from build123d import *

# Parameters (mm, degrees)
F0_R     = 8
F1_DEPTH = 3.5
F2_R     = 12.5
F2_R_2   = 8
F3_DEPTH = 1
F4_W     = 1.5
F4_H     = 2
F4_W_2   = 2
F4_H_2   = 1.5
F5_DEPTH = 0.25
F6_W     = 20
F6_H     = 2
F7_DEPTH = 1.5


with BuildPart() as f1:
    # F0 (on Top) → F1 (new body)
    with BuildSketch(Plane.XY):
        with BuildLine():
            ThreePointArc((0, -12.5), (8.838835, -8.838835), (12.5, 0))
            ThreePointArc((12.5, 0), (8.838835, 8.838835), (0, 12.5))
            ThreePointArc((0, 12.5), (-12.5, 0), (0, -12.5))
        make_face()
        Circle(F0_R, mode=Mode.SUBTRACT)
        with BuildLine():
            ThreePointArc((0, 12.5), (8.838835, 8.838835), (12.5, 0))
            ThreePointArc((12.5, 0), (8.838835, -8.838835), (0, -12.5))
            Line((0, -12.5), (35, -12.5))
            Line((35, -12.5), (116.388784, -2.506714))
            Line((116.388784, -2.506714), (116.388784, 2.506714))
            Line((116.388784, 2.506714), (35, 12.5))
            Line((35, 12.5), (0, 12.5))
        make_face()
    extrude(amount=F1_DEPTH)

    # F2 (on face) → F3 (join)
    with BuildSketch(Plane.XY.offset(3.5)):
        Circle(F2_R)
        Circle(F2_R_2, mode=Mode.SUBTRACT)
    extrude(amount=F3_DEPTH)

    # F4 (on face) → F5 (join)
    with BuildSketch(Plane.XY.offset(4.5)):
        with Locations((0, 10)):
            Rectangle(F4_W, F4_H)
        Polygon((-2.685895, 10.693384), (-4.112479, 10.229859), (-3.494445, 8.327746), (-2.067861, 8.791271), align=None)
        Polygon((-5.858875, 9.340026), (-7.072401, 8.458348), (-5.89683, 6.840314), (-4.683305, 7.721992), align=None)
        Polygon((-8.458348, 7.072401), (-9.340026, 5.858875), (-7.721992, 4.683305), (-6.840314, 5.89683), align=None)
        Polygon((-10.229859, 4.112479), (-10.693384, 2.685895), (-8.791271, 2.067861), (-8.327746, 3.494445), align=None)
        with Locations((-10, 0)):
            Rectangle(F4_W_2, F4_H_2)
        Polygon((-10.693384, -2.685895), (-10.229859, -4.112479), (-8.327746, -3.494445), (-8.791271, -2.067861), align=None)
        Polygon((-9.340026, -5.858875), (-8.458348, -7.072401), (-6.840314, -5.89683), (-7.721992, -4.683305), align=None)
        Polygon((-7.072401, -8.458348), (-5.858875, -9.340026), (-4.683305, -7.721992), (-5.89683, -6.840314), align=None)
        Polygon((-4.112479, -10.229859), (-2.685895, -10.693384), (-2.067861, -8.791271), (-3.494445, -8.327746), align=None)
        with Locations((0, -10)):
            Rectangle(F4_W, F4_H)
        Polygon((2.685895, -10.693384), (4.112479, -10.229859), (3.494445, -8.327746), (2.067861, -8.791271), align=None)
        Polygon((5.858875, -9.340026), (7.072401, -8.458348), (5.89683, -6.840314), (4.683305, -7.721992), align=None)
        Polygon((8.458348, -7.072401), (9.340026, -5.858875), (7.721992, -4.683305), (6.840314, -5.89683), align=None)
        Polygon((10.229859, -4.112479), (10.693384, -2.685895), (8.791271, -2.067861), (8.327746, -3.494445), align=None)
        with Locations((10, 0)):
            Rectangle(F4_W_2, F4_H_2)
        Polygon((10.693384, 2.685895), (10.229859, 4.112479), (8.327746, 3.494445), (8.791271, 2.067861), align=None)
        Polygon((9.340026, 5.858875), (8.458348, 7.072401), (6.840314, 5.89683), (7.721992, 4.683305), align=None)
        Polygon((7.072401, 8.458348), (5.858875, 9.340026), (4.683305, 7.721992), (5.89683, 6.840314), align=None)
        Polygon((4.112479, 10.229859), (2.685895, 10.693384), (2.067861, 8.791271), (3.494445, 8.327746), align=None)
    extrude(amount=F5_DEPTH)

    # F6 (on face) → F7 (cut)
    with BuildSketch(Plane.XY.offset(3.5)):
        with Locations((106.388784, -0.006714)):
            Rectangle(F6_W, F6_H)
    extrude(amount=-F7_DEPTH, mode=Mode.SUBTRACT)


solid = f1.part
Can you work these out from the model? Positions are in its coordinate system, mm. A direction names the side the tool comes from. Coordinates: 2 decimals unless noted, no trailing zeros. Write each loop counter-clockwise with the first axis right and the second up, starting at its lowest first coordinate (ties: lowest second). Pieces come first, ordered by that corner, then holes. Notation, with made-up numbers: (-23, 81.25) -> (22, 81.25) arc R9 cw to (22, 91.25) -> close; hole circle Ø2 at (42, -19). An arc over 180 degrees is marked (long way). Write each question's results on one line, items separated by ' | '. Start each with the question number.
Item 1: On a 3-axis mill with a long thin cutter (end or side, diameter ignored), from which of +Z, -Z, +X, -X, +Y, -Y can I reach the whole of each face in a straight line? I mean faces 1 (the cylindrical face through (-12.488, 0.55, 2.718)), 2 (the flat face through (106, 0, 2)), 3 (the flat face through (-3, 10, 4.75)). Say none if no direction works.
Item 2: If we section it at A-A, the plane x = 18: Write out the boundary of the cut face in (y, z).
Item 3: Please list where these lines run through material, in increasing order: probe 1 along Y at (x, z) = (0, 3.3); probe 2 along Z at (x, y) = (93, 3.5); probe 3 along X at (y, z) = (-2.25, 2.2).
Item 4: If we section it at B-B, the plane x = 92: Write out the boundary of the cut face in (y, z).
Item 5: Thinking about a two-plate mould opening in Y: for faces 4 (the flat face through (18, 12.5, 2)), 5 (the flat face through (-8, -6, 4.75)), 6 (the flat face through (-5, 7, 4.5)), which applies, released by +Y, released by -Y, zero draft, split by the parting line, or undercut?
Item 6: I'm going to push flat-ended pins straight in: P1, Ø1.6, axis at x = 103, z = 2.5, coming from the +Y side; P2, Ø1.2, axis at x = 110, z = 3, coming from the -Y side; P3, Ø1.5, axis at x = 102, z = 3, coming from the +Y side. Where does each tip first touch, or does it pass through?
Answer block:
1) face 1: +Z | face 2: +Z, +X | face 3: +Z, +X, -X, +Y, -Y
2) outline: (-12.5, 0) -> (12.5, 0) -> (12.5, 3.5) -> (-12.5, 3.5) -> close
3) probe 1: -12.5 to -8, 8 to 12.5 | probe 2: 0 to 3.5 | probe 3: -12.3 to -7.68, 7.68 to 116.39
4) outline: (-5.5, 0) -> (5.5, 0) -> (5.5, 3.5) -> (-5.5, 3.5) -> close
5) face 4: released by +Y | face 5: zero draft | face 6: undercut
6) P1: y = 4.25 | P2: y = -3.36 | P3: y = 4.37
